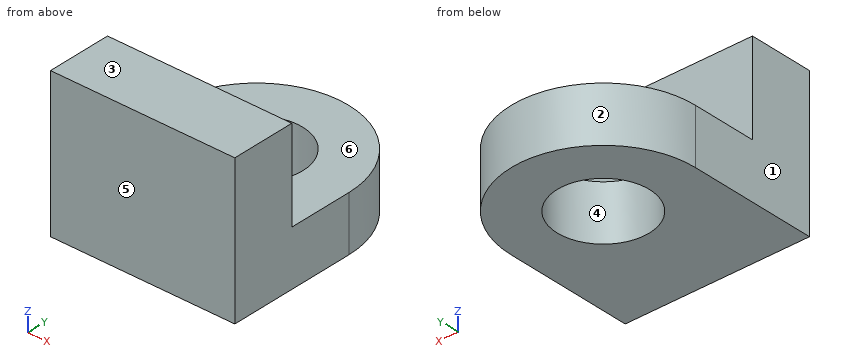
from build123d import *

# Parameters (mm, degrees)
F0_W     = 63.5
F0_H     = 44.45
F1_DEPTH = 19.05
F2_R     = 15.875
F3_DEPTH = 25.4
F4_W     = 63.5
F4_H     = 22.225
F5_DEPTH = 50.8


with BuildPart() as f1:
    # F0 (on Top) → F1 (new body)
    with BuildSketch(Plane.XY):
        Rectangle(F0_W, F0_H)
        with BuildLine():
            Line((-31.75, 22.225), (31.75, 22.225))
            ThreePointArc((31.75, 22.225), (0, 53.975), (-31.75, 22.225))
        make_face()
    extrude(amount=F1_DEPTH)

    # F2 (on face) → F3 (cut)
    with BuildSketch(Plane.XY.offset(19.05)):
        with Locations((0, 22.225)):
            Circle(F2_R)
    extrude(amount=-F3_DEPTH, mode=Mode.SUBTRACT)

    # F4 (on Top) → F5 (join)
    with BuildSketch(Plane.XY):
        with Locations((0, -11.1125)):
            Rectangle(F4_W, F4_H)
    extrude(amount=F5_DEPTH)


solid = f1.part
Read the model definition and answer for the solid it produces. Units are mm, in the model's axes. Face numbers are marked on the shaded views. A direction names the side the tool comes from. Round coordinates to 2 decimals unless told otherwise and drop trailing zeros. Write each loop counter-clockwise with the first axis right and the second up, starting at its lowest first coordinate (ties: lowest second). Pieces come first, ordered by that corner, then holes.
Q1. Find section A-A on x = 0. Determine the outline of the cut face in (y, z) (3 decimals).
Values:
outline: (-22.225, 0) - (6.35, 0) - (6.35, 19.05) - (0, 19.05) - (0, 50.8) - (-22.225, 50.8) - close; (38.1, 0) - (53.975, 0) - (53.975, 19.05) - (38.1, 19.05) - close
Q2. Find section D-D on x = 8.5. Determine the outline of the cut face in (y, z) (3 decimals), and give its area (3 significant figures).
Values:
outline: (-22.225, 0) - (8.817, 0) - (8.817, 19.05) - (0, 19.05) - (0, 50.8) - (-22.225, 50.8) - close; (35.633, 0) - (52.816, 0) - (52.816, 19.05) - (35.633, 19.05) - close
area: 1,620 mm2
Q3. Straight lines are drawn through the part: line 1 (Y direction, x = 0, z = 14.25) (3 decimals); line 2 (Y direction, x = 3, z = 26.5) (3 decimals); line 3 (Z direction, x = -9, y = 5). For each, find the intervals that lie inside material, in ascending order.
Values:
line 1: y = -22.225 to 6.35, 38.1 to 53.975
line 2: y = -22.225 to 0
line 3: z = 0 to 19.05
Q4. Find section B-B on y = 30. Determine the outline of the cut face in (x, z), and give its area (3 significant figures).
Values:
outline: (-30.78, 0) - (-13.84, 0) - (-13.84, 19.05) - (-30.78, 19.05) - close; (13.84, 0) - (30.78, 0) - (30.78, 19.05) - (13.84, 19.05) - close
area: 646 mm2
Q5. Flat-ended cylindrical pins translate along their axes: P1, Ø9.5, axis at x = 4.5, z = 38.5, coming from the +Y side; P2, Ø3, axis at x = 9.5, y = 33.5, coming from the +Z side; P3, Ø12, axis at y = 45, z = 8.5, coming from the +X side; P4, Ø3, axis at y = 13, z = 22.5, coming from the -X side. Find the tip coordinate at first contact, or state that the pin passes through.
Values:
P1: stops at y = 0
P2: stops at z = 19.05
P3: stops at x = 26.96
P4: passes through
Q6. Find section C-C on z = 36. Determine the outline of the cut face in (x, y) (3 decimals).
Values:
outline: (-31.75, -22.225) - (31.75, -22.225) - (31.75, 0) - (-31.75, 0) - close
Q7. A tool of negligible diameter and unlimited length cuts with its end or side. For the marked faces 5 and 6, from which of +Z, -Z, +X, -X, +Y, -Y can it reach the whole face along a straight path? Write none if from no direction.
Values:
face 5: +Z, -Z, +X, -X, -Y
face 6: +Z, +X, -X, +Y
Q8. The mould has two halves that part along X. Classify the marked faces 1, 2, 3 and 4: released by +X, released by -X, zero draft, split by the parting line, or undercut.
Values:
face 1: released by -X
face 2: split by the parting line
face 3: zero draft
face 4: undercut
